```python
from build123d import *

# Parameters (mm, degrees)
FILLET1_SIZE              = 1.27
FILLET1_SIZE_2            = 12.7
SKETCH3_W                 = 3.175
SKETCH3_H                 = 3.175
CUT_EXTRUDE1_DEPTH        = 46.228
F_4_40_TAPPED_HOLE1_D     = 2.2606
F_4_40_TAPPED_HOLE1_DEPTH = 7.62
F_4_40_TAPPED_HOLE1_TIP   = 0.679152758
CIRPATTERN1_COUNT         = 4
BOSS_EXTRUDE1_DEPTH       = 41.402


# Read off the part's stored shape, not the designer's step: #6-32 Tapped Hole1
with BuildPart() as part:
    # Sketch2 → Revolve1 (revolve)
    with BuildSketch(Plane.XY, mode=Mode.PRIVATE) as revolve1_sk:
        Polygon((50.8, 0), (-115.824, 0), (-115.824, 4.7625), (-103.124, 4.7625), (-103.124, 38.862), (-10.16, 38.862), (-9.525, 38.227), (-9.525, 38.862), (0, 38.862), (0, 17.4498), (4.572, 17.4498), (4.572, 6.35), (50.165, 6.35), (50.8, 5.715), align=None)
    revolve(revolve1_sk.sketch.rotate(Axis((88.99, 0, 0), (-1, 0, 0)), 90), axis=Axis((88.99, 0, 0), (-1, 0, 0)))

    # Fillet1
    # an asymmetric fillet: 12.7, 1.27 mm, written as the material it takes off along each edge
    with BuildSketch(Plane(origin=(-103.124, 0, 0), x_dir=(0, 0, -1), z_dir=(0, 1, 0))) as fillet1_piece_1:
        with BuildLine():
            Bezier((38.862 - FILLET1_SIZE, 0), (38.862, 0), (38.862, -FILLET1_SIZE_2), weights=[1, 0.707106781, 1])
            Line((38.862, -FILLET1_SIZE_2), (38.862, 0))
            Line((38.862, 0), (38.862 - FILLET1_SIZE, 0))
        make_face()
    revolve(axis=Axis((-103.124, 0, 0), (-1, 0, 0)), mode=Mode.SUBTRACT)

    # Sketch3 → Cut-Extrude1 (cut)
    with BuildSketch(Plane(origin=(50.8, 0, 0), x_dir=(0, 0, -1), z_dir=(1, 0, 0))):
        with Locations((0, 6.35)):
            Rectangle(SKETCH3_W, SKETCH3_H)
    extrude(amount=-CUT_EXTRUDE1_DEPTH, mode=Mode.SUBTRACT)

    # Sketch8 → #8-32 Tapped Hole3 (revolve, cut)
    with BuildSketch(Plane(origin=(0, 0, -25), x_dir=(0, 0, -1), z_dir=(0, 1, 0))):
        Polygon((0, 0), (0, 11.705806461), (1.7272, 10.668), (1.7272, 0), align=None)
    f_8_32_tapped_hole3 = revolve(axis=Axis((6.35, 0, -25), (-1, 0, 0)), mode=Mode.SUBTRACT)

    # #6-32 Tapped Hole1 outline → #6-32 Tapped Hole1 (revolve, cut)
    with BuildSketch(Plane(origin=(0, 19.813624417, 28.296788218), x_dir=(0, 1, 0), z_dir=(0, 0, -1))):
        Polygon((1.35255, -93.726), (0, -92.91330597), (0, -103.124), (1.35255, -103.124), align=None)
    f_6_32_tapped_hole1 = revolve(axis=Axis((0, 19.813624417, 28.296788218), (1, 0, 0)), mode=Mode.SUBTRACT)

    # #4-40 Tapped Hole1
    with Locations(Plane.ZY.offset(103.124)):
        with Locations((-23, 0), (23, 0)):
            Hole(F_4_40_TAPPED_HOLE1_D / 2, depth=F_4_40_TAPPED_HOLE1_DEPTH)
            with Locations((0, 0, -(F_4_40_TAPPED_HOLE1_DEPTH + F_4_40_TAPPED_HOLE1_TIP / 2))):  # 118° drill point
                Cone(0, F_4_40_TAPPED_HOLE1_D / 2, F_4_40_TAPPED_HOLE1_TIP, mode=Mode.SUBTRACT)

    # CirPattern1: #8-32 Tapped Hole3, #6-32 Tapped Hole1 ×4 about axis
    cirpattern1_axis = Axis((0, 0, 0), (1, 0, 0))
    add([f_8_32_tapped_hole3.rotate(cirpattern1_axis, i * 360 / CIRPATTERN1_COUNT) for i in range(1, CIRPATTERN1_COUNT)], mode=Mode.SUBTRACT)
    add([f_6_32_tapped_hole1.rotate(cirpattern1_axis, i * 360 / CIRPATTERN1_COUNT) for i in range(1, CIRPATTERN1_COUNT)], mode=Mode.SUBTRACT)

    # Sketch12 → Boss-Extrude1 (add)
    with BuildSketch(Plane(origin=(0, 0, 0), x_dir=(1, 0, 0), z_dir=(0, 1, 0))):
        with BuildLine():
            Line((-92.964, -5.08), (-82.804, -5.08))
            ThreePointArc((-82.804, -5.08), (-77.724, 0), (-82.804, 5.08))
            Line((-82.804, 5.08), (-92.964, 5.08))
            Line((-92.964, 5.08), (-92.964, -5.08))
        make_face()
    extrude(amount=BOSS_EXTRUDE1_DEPTH)


solid = part.part
```
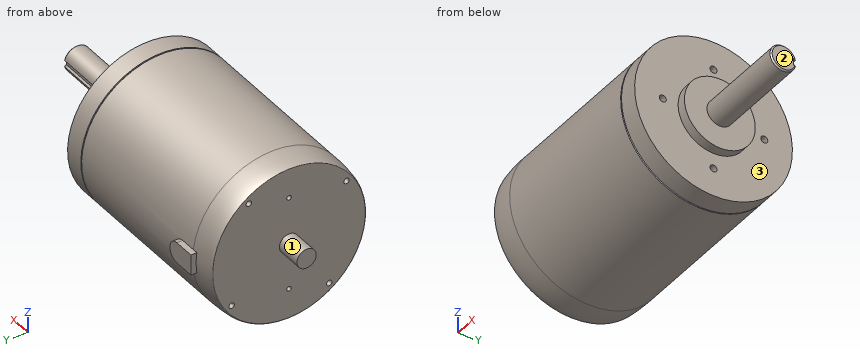
Could you check a few things on this model? Use its own coordinates, in mm. Face numbers are marked on the shaded views. A direction names the side the tool comes from. Round coordinates to 2 decimals unless told otherwise and drop trailing zeros. Loops run counter-clockwise (first coordinate to the right, second up) from the corner with the lowest first, then second, coordinate; pieces in that order, holes last. Notation, with made-up numbers: (70, 80.5) - (95, 80.5) arc R11 cw to (95, 95.5) - close; hole circle Ø4 at (64.5, -1). An arc over 180 degrees is marked (long way). Answer as CSV lines item,"result".
1. Please list where these lines run through material, in increasing order: line 1 along Z through (x, y) = (-97.25, 0); line 2 along Z through (x, y) = (-100.75, 0); line 3 along X through (y, z) = (-21.5, -16). Write a range as [from, to].
Filled in:
line 1,"z = [-38.66, -24.13], [-21.87, 21.87], [24.13, 38.66]"
line 2,"z = [-38.33, -24.13], [-21.87, 21.87], [24.13, 38.33]"
line 3,"x = [-103.12, 0]"
2. I want a section at B-B on x = -57.5. List the corners of the cut face in (y, z) for me, then the cut area to 3 significant figures.
Filled in:
outline,"circle Ø77.72 at (0, 0)"
area,"4,740 mm^2"
3. I want a section at C-C on x = -99. Count the separate pieces of the cut face and the enclosed holes in it, then the cut area to 3 significant figures.
Filled in:
separate pieces,"1"
enclosed holes,"6"
area,"4,630 mm^2"
4. On a 3-axis mill with a long thin cutter (end or side, diameter ignored), from which of +Z, -Z, +X, -X, +Y, -Y can I reach the whole of each face in a straight line? I mean the marked faces 1, 2 and 3. Say none if no direction works.
Filled in:
face 1,"-X"
face 2,"+Z, -Z, +X, +Y, -Y"
face 3,"+X"
5. For pin 1 Ø3.5 at (y, z) = (19.81, 28.3) entering from +X; pin 2 Ø3.5 at (x, z) = (33, 0) entering from +Y; pin 3 Ø3 at (x, z) = (-3, 27.5) entering from -Y, each with a flat end and sliding along its axis, tell me the tip position at first contact or that it passes through.
Filled in:
pin 1,"stops at x = 0"
pin 2,"stops at y = 6.15"
pin 3,"stops at y = -28.88"
6. I want a section at A-A on x = -5. List the corners of the cut face in (y, z) for me, then the cut area to 3 significant figures.
Filled in:
outline,"circle Ø77.72 at (0, 0); hole circle Ø3.45 at (-25, 0); hole circle Ø3.45 at (0, -25); hole circle Ø3.45 at (0, 25); hole circle Ø3.45 at (25, 0)"
area,"4,710 mm^2"
